Study the drawing (mm; zero at the part's minimum x, y, z) and answer. A direction names the side the tool comes from. Coordinates: 2 decimals unless noted, no trailing zeros. Loops run counter-clockwise (first coordinate to the right, second up) from the corner with the lowest first, then second, coordinate; pieces in that order, holes last. Notation, with made-up numbers: (-16, 72.25) -> (19, 72.25) arc R24 ccw to (19, 82.25) -> close; hole circle Ø10 at (63.25, 4.25). An arc over 180 degrees is marked (long way). Answer in a Markdown table with one row per item.
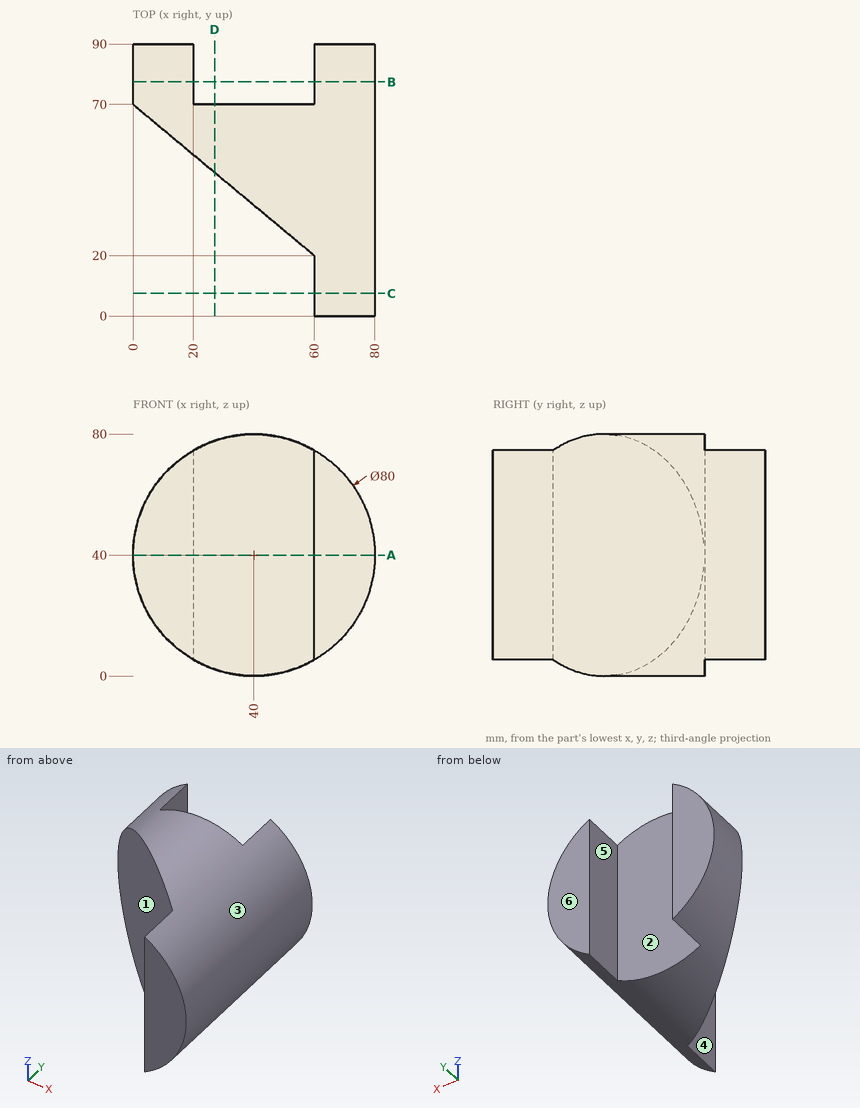
1. Find the intervals of material crossed by probe 1 along X at (y, z) = (80, 28.5); probe 2 along Z at (x, y) = (44, 35.5); probe 3 along Z at (x, y) = (67.5, 6), in increasing order.
A:
| item | result |
|---|---|
| probe 1 | x = 1.69 to 20, 60 to 78.31 |
| probe 2 | z = 0.2 to 79.8 |
| probe 3 | z = 10.95 to 69.05 |
2. A tool of negligible diameter and unlimited length cuts with its end or side. For the marked faces 4, 5 and 6, from which of +Z, -Z, +X, -X, +Y, -Y can it reach the whole face along a straight path? Write none if from no direction.
A:
| item | result |
|---|---|
| face 4 | +Z, -Z, -X, -Y |
| face 5 | +Z, -Z, +Y |
| face 6 | +Z, -Z, +X, -X, +Y |
3. The mould has two halves that part along X. Classify the marked faces 1, 2 and 3: pulls with the +X half, pulls with the -X half, needs draft (parallel to the pull), parting line crosses it, or undercut.
A:
| item | result |
|---|---|
| face 1 | pulls with the -X half |
| face 2 | undercut |
| face 3 | parting line crosses it |
4. Given pin 1 Ø22 at (y, z) = (5.5, 42) entering from -X; pin 2 Ø6 at (y, z) = (79, 30.5) entering from +X; pin 3 Ø1.5 at (y, z) = (17, 66.5) entering from +X, each flat-ended and moving along its own axis, determine where each tip first touches the part or whether it passes through.
A:
| item | result |
|---|---|
| pin 1 | stops at x = 60 |
| pin 2 | stops at x = 79.47 |
| pin 3 | stops at x = 70.61 |
5. A cutting plane is placed at C-C on y = 7.5. Give the vertices of the cut face in (x, z), and give its area (3 significant figures).
A:
| item | result |
|---|---|
| outline | (60, 5.36) arc R40 ccw to (60, 74.64) -> close |
| area | 983 mm2 |
6. A cutting plane is placed at D-D on x = 27. Give the vertices of the cut face in (y, z), and give its area (3 significant figures).
A:
| item | result |
|---|---|
| outline | (47.5, 2.17) -> (70, 2.17) -> (70, 77.83) -> (47.5, 77.83) -> close |
| area | 1,700 mm2 |
7. A cutting plane is placed at B-B on y = 77.5. Give the vertices of the cut face in (x, z).
A:
| item | result |
|---|---|
| outline | (20, 5.36) -> (20, 74.64) arc R40 ccw to start; (60, 5.36) arc R40 ccw to (60, 74.64) -> close |
8. A cutting plane is placed at A-A on z = 40. Give the vertices of the cut face in (x, y), and give its area (3 significant figures).
A:
| item | result |
|---|---|
| outline | (0, 70) -> (60, 20) -> (60, 0) -> (80, 0) -> (80, 90) -> (60, 90) -> (60, 70) -> (20, 70) -> (20, 90) -> (0, 90) -> close |
| area | 3,700 mm2 |
